Part model, mm, in its own coordinate system. A direction names the side the tool comes from. Round coordinates to 2 decimals unless told otherwise and drop trailing zeros. Write each loop counter-clockwise with the first axis right and the second up, starting at its lowest first coordinate (ties: lowest second). Pieces come first, ordered by that corner, then holes. Notation, with made-up numbers: (-39, -19.75) -> (-5, -19.75) arc R23 ccw to (-5, 17.25) -> close; hole circle Ø7 at (60.5, 15). An arc over 180 degrees is marked (long way). Use CSV: the item, a comma, the result in double quotes. Start each with the question number.
(1) Which spindle directions (+Z, -Z, +X, -X, +Y, -Y) get a long thin tool onto all of the face, cutting with end or side? Do faces 4 (the flat face through (6, 12, 6)), 5 (the flat face through (6, 89, 0)), 6 (the flat face through (0, -11, 0)). Say none if no direction does.
(2) Two-plate mould, pull along Y, no slides. Class faces 1 (the cylindrical face through (-7.493, -5.423, -0.33)), 2 (the flat face through (6, 47, 0)), 3 (the flat face through (-4, 0, -7)): released by +Y, released by -Y, zero draft, split by the parting line, or undercut.
(3) Saw through at D-D (y = 3.5). Give the cut face in (x, z).
(4) Drop flat-ended pins along their axis: pin 1 (13.5 mm diameter, centred on y = 78, z = 1, fed in from +X); pin 2 (12 mm diameter, centred on y = 26.5, z = -7, fed in from -X); pin 3 (2 mm diameter, centred on x = -1.5, y = 56.5, fed in from +Z). Give the stop position or say it passes through.
(5) Saw through at B-B (z = 0). Give the cut face in (x, y), plus the area to 3 significant figures.
(6) Saw through at C-C (x = 6.5). Give the cut face in (y, z), plus the area to 3 significant figures.
(7) Probe line 1 (Y direction, x = 6.5, z = 3); line 2 (Y direction, x = 7.5, z = 3.75); line 3 (X direction, y = 71, z = 0.5). List the from-to ranges inside material, lowest first. Write a range as [from, to].
(8) Saw through at A-A (x = 0). Give the cut face in (y, z).
```python
from build123d import *

# Parameters (mm, degrees)
SKETCH1_R           = 7.5
BOSS_EXTRUDE1_DEPTH = 11
SKETCH2_R           = 15
BOSS_EXTRUDE2_DEPTH = 12
SKETCH3_R           = 8
BOSS_EXTRUDE3_DEPTH = 80
SKETCH4_W           = 9.801818504
SKETCH4_H           = 42
CUT_EXTRUDE1_DEPTH  = 40


with BuildPart() as part:
    # Sketch1 → Boss-Extrude1 (new body)
    with BuildSketch(Plane(origin=(0, 0, 0), x_dir=(1, 0, 0), z_dir=(0, 1, 0))):
        Circle(SKETCH1_R)
    extrude(amount=-BOSS_EXTRUDE1_DEPTH)

    # Sketch2 → Boss-Extrude2 (add)
    with BuildSketch(Plane(origin=(0, 0, 0), x_dir=(1, 0, 0), z_dir=(0, 1, 0))):
        Circle(SKETCH2_R)
    extrude(amount=BOSS_EXTRUDE2_DEPTH)

    # Sketch3 → Boss-Extrude3 (add)
    with BuildSketch(Plane(origin=(0, 12, 0), x_dir=(1, 0, 0), z_dir=(0, 1, 0))):
        Circle(SKETCH3_R)
    extrude(amount=BOSS_EXTRUDE3_DEPTH)

    # Sketch4 → Cut-Extrude1 (cut, symmetric)
    with BuildSketch(Plane.XY):
        with Locations((9.900909252, 68)):
            Rectangle(SKETCH4_W, SKETCH4_H)
    extrude(amount=CUT_EXTRUDE1_DEPTH, both=True, mode=Mode.SUBTRACT)


solid = part.part
```
Answers:
1,face 4,"+Y"
1,face 5,"+Z, -Z, +X"
1,face 6,"+Z, -Z, +X, -X, -Y"
2,face 1,"zero draft"
2,face 2,"undercut"
2,face 3,"released by -Y"
3,outline,"circle Ø30 at (0, 0)"
4,pin 1,"stops at x = 5"
4,pin 2,"stops at x = -7.94"
4,pin 3,"stops at z = 7.98"
5,outline,"(-15, 0) -> (-7.5, 0) -> (-7.5, -11) -> (7.5, -11) -> (7.5, 0) -> (15, 0) -> (15, 12) -> (8, 12) -> (8, 47) -> (5, 47) -> (5, 89) -> (8, 89) -> (8, 92) -> (-8, 92) -> (-8, 12) -> (-15, 12) -> close"
5,area,"1,680 mm²"
6,outline,"(-11, -3.74) -> (0, -3.74) -> (0, -13.52) -> (12, -13.52) -> (12, -4.66) -> (47, -4.66) -> (47, 4.66) -> (12, 4.66) -> (12, 13.52) -> (0, 13.52) -> (0, 3.74) -> (-11, 3.74) -> close; (89, -4.66) -> (92, -4.66) -> (92, 4.66) -> (89, 4.66) -> close"
6,area,"761 mm²"
7,line 1,"y = [-11, 47], [89, 92]"
7,line 2,"y = [0, 12]"
7,line 3,"x = [-7.98, 5]"
8,outline,"(-11, -7.5) -> (0, -7.5) -> (0, -15) -> (12, -15) -> (12, -8) -> (92, -8) -> (92, 8) -> (12, 8) -> (12, 15) -> (0, 15) -> (0, 7.5) -> (-11, 7.5) -> close"
